Check sheet for the drawn part. Datum: minimum x, y, z corner. Units: mm. A direction names the side the tool comes from. Give positions to 0.01 mm unless a question says otherwise; leave off trailing zeros. Order: outer loops, then holes, each group sorted by start corner. A loop starts at its lowest first (then second) coordinate and runs counter-clockwise, first axis right, second up. Notation, with made-up numbers: M 20,-26.75 L 40,-26.75 A10 cw 40,-15.75 Z; hole C 23,55.25 d8. An arc over 180 degrees is marked long. Answer as CSV lines item,"result". Start each with the question number.
Q1. Section check B-B, the plane x = 8.75. Record the boundary of the cut face in (y, z).
Q2. Section check A-A, the plane y = 7. Record the boundary of the cut face in (x, z), then the cut area to 3 significant figures.
Q3. Go/stop test with flat-tipped pins: pin 1 (1 mm diameter, centred on y = 10.5, z = 1.5, fed in from -X); pin 2 (0.5 mm diameter, centred on y = 11.5, z = 3, fed in from +X); pin 3 (3 mm diameter, centred on y = 3, z = 2.5, fed in from +X). Record where each tip stops, or that it passes through.
Q4. Mould release check, pull along Y, two halves, no side actions. Record for the marked faces 1, 2, 3 and 4: +Y half, -Y half, draft (parallel to the pull), parting line (faces both ways), or undercut.
Q5. Set-up check for the marked faces 5 and 6: record each of +Z, -Z, +X, -X, +Y, -Y from which the full face is reachable in a straight line by a thin tool's end or side.
Q6. Section check D-D, the plane x = 7. Record the boundary of the cut face in (y, z).
Q7. Section check C-C, the plane z = 1.1. Record the boundary of the cut face in (x, y).
Q8. Thickness scan on line 1 (X direction, y = 7, z = 2.3); line 2 (Y direction, x = 7, z = 3.25); line 3 (Z direction, x = 0.5, y = 5). Record the ranges inside material, lowest first.
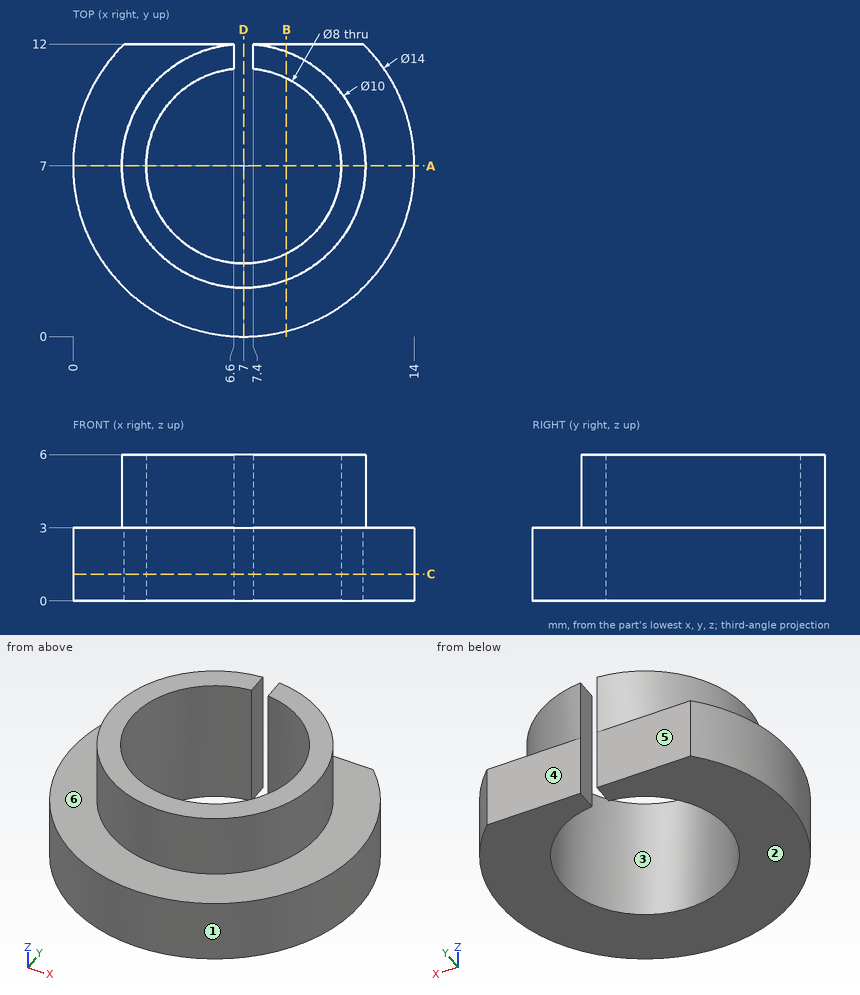
Answer block:
1,outline,"M 0.22,0 L 3.4,0 L 3.4,6 L 2.32,6 L 2.32,3 L 0.22,3 Z; M 10.6,0 L 12,0 L 12,3 L 11.68,3 L 11.68,6 L 10.6,6 Z"
2,outline,"M 0,0 L 3,0 L 3,6 L 2,6 L 2,3 L 0,3 Z; M 11,0 L 14,0 L 14,3 L 12,3 L 12,6 L 11,6 Z"
2,area,"24.0 mm2"
3,pin 1,"stops at x = 0.68"
3,pin 2,"stops at x = 12.56"
3,pin 3,"stops at x = 13.54"
4,face 1,"parting line"
4,face 2,"draft"
4,face 3,"undercut"
4,face 4,"+Y half"
5,face 5,"+Z, -Z, +X, -X, +Y"
5,face 6,"+Z"
6,outline,"M 0,0 L 3,0 L 3,6 L 2,6 L 2,3 L 0,3 Z"
7,outline,"M 2.1,12 A7 ccw long 11.9,12 L 7.4,12 L 7.4,10.98 A4 cw long 6.6,10.98 L 6.6,12 Z"
8,line 1,"x = 0 to 3, 11 to 14"
8,line 2,"y = 2 to 3"
8,line 3,"z = 0 to 3"
